from build123d import *

# Parameters (mm, degrees)
SKIZZE1_R                       = 1.25
SKIZZE1_R_2                     = 5
AUFSATZ_LINEAR_AUSTRAGEN1_DEPTH = 0.825
VERRUNDUNG1_R                   = 1.5


with BuildPart() as part:
    # Skizze1 → Aufsatz-Linear austragen1 (new body, symmetric)
    with BuildSketch(Plane(origin=(0, 0, 0), x_dir=(1, 0, 0), z_dir=(0, 1, 0))):
        Polygon((-13.3, -6), (-13.3, -11.6), (-6, -11.6), (-6, -13.3), (6, -13.3), (6, -11.6), (13.3, -11.6), (13.3, -6), (15, -6), (15, 6), (13.3, 6), (13.3, 11.6), (6, 11.6), (6, 13.3), (-6, 13.3), (-6, 11.6), (-13.3, 11.6), (-13.3, 6), (-15, 6), (-15, -6), align=None)
        with Locations((0, -8)):
            Circle(SKIZZE1_R, mode=Mode.SUBTRACT)
        with Locations((0, 8)):
            Circle(SKIZZE1_R, mode=Mode.SUBTRACT)
        Circle(SKIZZE1_R_2, mode=Mode.SUBTRACT)
    extrude(amount=AUFSATZ_LINEAR_AUSTRAGEN1_DEPTH, both=True)

    # Verrundung1
    verrundung1_edges = [part.edges().sort_by_distance(p)[0] for p in [
        (-6, 0, 11.6),
        (-13.3, 0, 6),
        (-13.3, 0, -6),
        (-6, 0, -11.6),
        (6, 0, -11.6),
        (13.3, 0, -6),
        (13.3, 0, 6),
        (6, 0, 11.6),
    ]]
    fillet(verrundung1_edges, radius=VERRUNDUNG1_R)


solid = part.part
Input: part model. Units: mm. Frame: model coordinates. A direction names the side the tool comes from. Give positions to 0.01 mm unless a question says otherwise; leave off trailing zeros. Loops run counter-clockwise (first coordinate to the right, second up) from the corner with the lowest first, then second, coordinate; pieces in that order, holes last. Notation, with made-up numbers: (30, 19) -> (89, 19) arc R4 ccw to (89, 26) -> close; hole circle Ø6 at (-28.5, -38.5). An arc over 180 degrees is marked (long way). Answer as a JSON object with one key per item and string values. Group by question number.
Item 1: Cut plane D-D, the plane z = -8. Return the cut outline in (x, y) (3 decimals), and give its area (3 significant figures).
Item 2: Pull-direction query (Z, two-part tool) for faces 6 (the flat face through (10, 0, -11.6)), 7 (the cylindrical face through (-0.27, -0.01, -6.78)), 8 (the cylindrical face through (-13.73, -0.01, 6.45)); classes: released by +Z, released by -Z, zero draft, split by the parting line, or undercut.
Item 3: Cut plane A-A, the plane x = 0. Return the cut outline in (y, z) (3 decimals), and give its area (3 significant figures).
Item 4: Cut plane C-C, the plane y = 0.15. State how many separate pieces and enclosed holes the cut face has, and give its area (3 significant figures).
Item 5: Pin query (flat end, axial travel): P1, Ø0.8, axis at y = 0, z = 9, coming from the -X side; P2, Ø0.8, axis at x = -10, y = -0.5, coming from the -Z side; P3, Ø0.5, axis at y = 0, z = -8.5, coming from the +X side; P4, Ø13, axis at x = 0, z = 0, coming from the -Y side (3 decimals). Return the tip coordinate at first contact, or that it passes through.
Item 6: Line query: probe 1 along Z at (x, y) = (0, -0.35); probe 2 along X at (y, z) = (0, 0); probe 3 along Z at (x, y) = (0.5, 0.35). Output: solid intervals per line, ascending.
Item 7: Reachability of faces 1 (the flat face through (-13.3, 0, -10)), 2 (the flat face through (-10, 0, 11.6)), 3 (the flat face through (0, 0.825, 6)), 4 (the flat face through (13.3, 0, -10)), 5 (the flat face through (10, 0, 11.6)) from +Z, -Z, +X, -X, +Y, -Y: full face, straight path, thin tool, end or side. Return the list, or none.
Item 8: Cut plane B-B, the plane z = 0. Return the cut outline in (x, y) (3 decimals), and give its area (3 significant figures).
Checks:
{
 "1": {"outline": "(-13.3, -0.825) -> (-1.25, -0.825) -> (-1.25, 0.825) -> (-13.3, 0.825) -> close; (1.25, -0.825) -> (13.3, -0.825) -> (13.3, 0.825) -> (1.25, 0.825) -> close", "area": "39.8 mm²"},
 "2": {"face 6": "released by -Z", "face 7": "undercut", "face 8": "released by +Z"},
 "3": {"outline": "(-0.825, -13.3) -> (0.825, -13.3) -> (0.825, -9.25) -> (-0.825, -9.25) -> close; (-0.825, -6.75) -> (0.825, -6.75) -> (0.825, -5) -> (-0.825, -5) -> close; (-0.825, 5) -> (0.825, 5) -> (0.825, 6.75) -> (-0.825, 6.75) -> close; (-0.825, 9.25) -> (0.825, 9.25) -> (0.825, 13.3) -> (-0.825, 13.3) -> close", "area": "19.1 mm²"},
 "4": {"separate pieces": "1", "enclosed holes": "3", "area": "614 mm²"},
 "5": {"P1": "stops at x = -13.3", "P2": "stops at z = -11.6", "P3": "stops at x = 13.3", "P4": "stops at y = -0.825"},
 "6": {"probe 1": "z = -13.3 to -9.25, -6.75 to -5, 5 to 6.75, 9.25 to 13.3", "probe 2": "x = -15 to -5, 5 to 15", "probe 3": "z = -13.3 to -9.15, -6.85 to -4.97, 4.97 to 6.85, 9.15 to 13.3"},
 "7": {"face 1": "-Z, -X, +Y, -Y", "face 2": "+Z, -X, +Y, -Y", "face 3": "+Z, -Z, +X, -X, +Y", "face 4": "-Z, +X, +Y, -Y", "face 5": "+Z, +X, +Y, -Y"},
 "8": {"outline": "(-15, -0.825) -> (-5, -0.825) -> (-5, 0.825) -> (-15, 0.825) -> close; (5, -0.825) -> (15, -0.825) -> (15, 0.825) -> (5, 0.825) -> close", "area": "33.0 mm²"}
}
